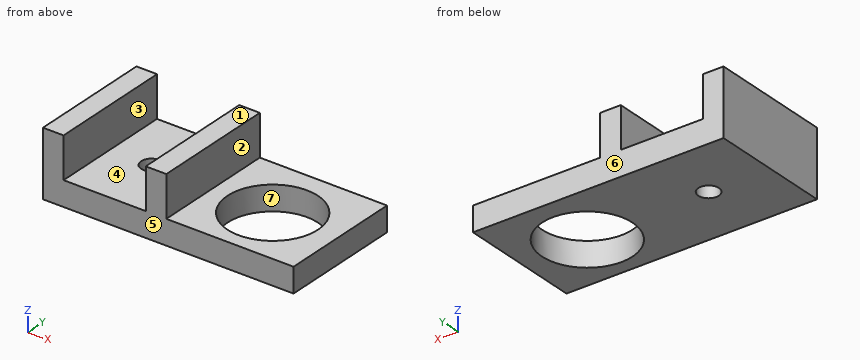
```python
from build123d import *

# Parameters (mm, degrees)
F0_W     = 5
F0_H     = 10
F1_DEPTH = 30
F3_D     = 22
F5_D     = 5


# Not quite as in the source:
# - a feature names something its author has since deleted; it is built from what else it names


with BuildPart() as f1:
    # F0 (on Front) → F1 (new body)
    with BuildSketch(Plane.XZ):
        with Locations((-33.2201862009, 15.0932593657)):
            Rectangle(F0_W, F0_H)
        Polygon((-30.7201862009, 10.0932593657), (-35.7201862009, 10.0932593657), (-35.7201862009, 4.0932593657), (25.2284052642, 4.0932593657), (25.2284052642, 10.0932593657), (-5.7201862009, 10.0932593657), (-10.7201862009, 10.0932593657), align=None)
        with Locations((-8.2201862009, 15.0932593657)):
            Rectangle(F0_W, F0_H)
    extrude(amount=F1_DEPTH)

    # F3 (through all)
    with Locations(Plane.XY.offset(10.0932593657)):
        with Locations((9.2798137991, -15.640585908)):
            Hole(F3_D / 2)

    # F5 (through all)
    with Locations(Plane.XY.offset(10.0932593657)):
        with Locations((-20.7201862009, -15)):
            Hole(F5_D / 2)


solid = f1.part
```
Verification items for the finished model (mm, model axes). Face numbers are marked on the shaded views. A direction names the side the tool comes from. Coordinates: 2 decimals unless noted, no trailing zeros. Write each loop counter-clockwise with the first axis right and the second up, starting at its lowest first coordinate (ties: lowest second). Pieces come first, ordered by that corner, then holes. Notation, with made-up numbers: M -25,0.5 L 13,0.5 A17 cw 13,11.5 Z; hole C 26.25,56 d6. An arc over 180 degrees is marked long. Answer as a JSON object with one key per item and string values. Group by question number.
(1) Tool access check on the marked faces 1, 2 and 3. Record the directions out of +Z, -Z, +X, -X, +Y, -Y that give a thin tool (end or side, any length) a straight path to the whole face; none if there is none.
(2) Material ranges on line 1 (X direction, y = -25.5, z = 10.25); line 2 (X direction, y = -16.5, z = 6); line 3 (Z direction, x = -4, y = -9), recorded low to high.
(3) Gauge pin test, flat ends, axial feed: pin 1 (3 mm diameter, centred on x = -4, z = 15, fed in from +Y); pin 2 (6 mm diameter, centred on x = 5, y = -26, fed in from +Z); pin 3 (3 mm diameter, centred on y = -20.5, z = 14.5, fed in from +X). Record the tip position at first contact, or that the pin passes through.
(4) Cross-section at B-B, the plane y = -7.75. Record the cut outline in (x, z), and give its area (3 significant figures).
(5) Release check for a two-part mould opening along Y. For the marked faces 4, 5, 6 and 7 record: +Y half, -Y half, draft (parallel to the pull), parting line (faces both ways), or undercut.
(6) Cross-section at A-A, the plane z = 13.5. Record the cut outline in (x, y), and give its area (3 significant figures).
(7) Cross-section at D-D, the plane y = -15. Record the cut outline in (x, z), and give its area (3 significant figures).
(8) Cross-section at C-C, the plane x = 11.5. Record the cut outline in (y, z).
Reply:
{
 "1": {"face 1": "+Z, +X, -X, +Y, -Y", "face 2": "+Z, +X, +Y, -Y", "face 3": "+Z, +Y, -Y"},
 "2": {"line 1": "-35.72 to -30.72, -10.72 to -5.72", "line 2": "-35.72 to -22.72, -18.72 to -1.69, 20.25 to 25.23", "line 3": "4.09 to 10.09"},
 "3": {"pin 1": "through", "pin 2": "z = 10.09", "pin 3": "x = -5.72"},
 "4": {"outline": "M -35.72,4.09 L 1.62,4.09 L 1.62,10.09 L -5.72,10.09 L -5.72,20.09 L -10.72,20.09 L -10.72,10.09 L -30.72,10.09 L -30.72,20.09 L -35.72,20.09 Z; M 16.94,4.09 L 25.23,4.09 L 25.23,10.09 L 16.94,10.09 Z", "area": "374 mm²"},
 "5": {"face 4": "draft", "face 5": "-Y half", "face 6": "+Y half", "face 7": "undercut"},
 "6": {"outline": "M -35.72,-30 L -30.72,-30 L -30.72,0 L -35.72,0 Z; M -10.72,-30 L -5.72,-30 L -5.72,0 L -10.72,0 Z", "area": "300 mm²"},
 "7": {"outline": "M -35.72,4.09 L -23.22,4.09 L -23.22,10.09 L -30.72,10.09 L -30.72,20.09 L -35.72,20.09 Z; M -18.22,4.09 L -1.7,4.09 L -1.7,10.09 L -5.72,10.09 L -5.72,20.09 L -10.72,20.09 L -10.72,10.09 L -18.22,10.09 Z; M 20.26,4.09 L 25.23,4.09 L 25.23,10.09 L 20.26,10.09 Z", "area": "304 mm²"},
 "8": {"outline": "M -30,4.09 L -26.41,4.09 L -26.41,10.09 L -30,10.09 Z; M -4.87,4.09 L 0,4.09 L 0,10.09 L -4.87,10.09 Z"}
}
